```python
from build123d import *

# Parameters (mm, degrees)
BOSS_EXTRU_1_DEPTH      = 600
ESQUISSE2_R             = 15
ENL_V_MAT_EXTRU_1_DEPTH = 607.630035524


with BuildPart() as part:
    # Esquisse1 → Boss.-Extru.1 (new body)
    with BuildSketch(Plane.XY):
        with BuildLine():
            Line((2, -2), (78, -2))
            ThreePointArc((78, -2), (79.414213562, -1.414213562), (80, 0))
            Line((80, 0), (80, 36))
            ThreePointArc((80, 36), (79.414213562, 37.414213562), (78, 38))
            Line((78, 38), (2, 38))
            ThreePointArc((2, 38), (0.585786438, 37.414213562), (0, 36))
            Line((0, 36), (0, 0))
            ThreePointArc((0, 0), (0.585786438, -1.414213562), (2, -2))
        make_face()
        with BuildLine():
            Line((4, 4), (4, 32))
            ThreePointArc((4, 32), (4.585786438, 33.414213562), (6, 34))
            Line((6, 34), (74, 34))
            ThreePointArc((74, 34), (75.414213562, 33.414213562), (76, 32))
            Line((76, 32), (76, 4))
            ThreePointArc((76, 4), (75.414213562, 2.585786438), (74, 2))
            Line((74, 2), (6, 2))
            ThreePointArc((6, 2), (4.585786438, 2.585786438), (4, 4))
        make_face(mode=Mode.SUBTRACT)
    extrude(amount=BOSS_EXTRU_1_DEPTH)

    # Esquisse2 → Enlèv. mat.-Extru.1 (cut, through all)
    with BuildSketch(Plane(origin=(0, 38, 0), x_dir=(1, 0, 0), z_dir=(0, 1, 0))):
        with Locations(Location((40, -300, 0), (0, 0, 180))):
            Circle(ESQUISSE2_R)
    extrude(amount=-ENL_V_MAT_EXTRU_1_DEPTH, mode=Mode.SUBTRACT)


solid = part.part
```
Could you check a few things on this model? Use its own coordinates, in mm. A direction names the side the tool comes from. Round coordinates to 2 decimals unless told otherwise and drop trailing zeros. Write each loop counter-clockwise with the first axis right and the second up, starting at its lowest first coordinate (ties: lowest second). Pieces come first, ordered by that corner, then holes.
(1) Suppose I cut it at B-B on z = 300. Write out the boundary of the cut face in (x, y), and give its area (3 significant figures).
Findings below:
outline: (0, 0) arc R2 ccw to (2, -2) - (25, -2) - (25, 2) - (6, 2) arc R2 cw to (4, 4) - (4, 32) arc R2 cw to (6, 34) - (25, 34) - (25, 38) - (2, 38) arc R2 ccw to (0, 36) - close; (55, -2) - (78, -2) arc R2 ccw to (80, 0) - (80, 36) arc R2 ccw to (78, 38) - (55, 38) - (55, 34) - (74, 34) arc R2 cw to (76, 32) - (76, 4) arc R2 cw to (74, 2) - (55, 2) - close
area: 656 mm2
(2) Suppose I cut it at A-A on y = 25.5. Write out the boundary of the cut face in (x, z).
Findings below:
outline: (0, 0) - (4, 0) - (4, 600) - (0, 600) - close; (76, 0) - (80, 0) - (80, 600) - (76, 600) - close
(3) Thinking about a two-plate mould opening in Y: for faces 1 (the face through (23, -2, 296)), 2 (the face through (24, 38, 296)), 3 (the face through (41.953, 0.028, 314.872)), 4 (the face through (55, 34, 296)), which applies, +Y half, -Y half, draft (parallel to the pull), parting line (faces both ways), or undercut?
Findings below:
face 1: -Y half
face 2: +Y half
face 3: draft
face 4: undercut
(4) Suppose I cut it at D-D on z = 52.5. Write out the boundary of the cut face in (x, y), and give its area (3 significant figures).
Findings below:
outline: (0, 0) arc R2 ccw to (2, -2) - (78, -2) arc R2 ccw to (80, 0) - (80, 36) arc R2 ccw to (78, 38) - (2, 38) arc R2 ccw to (0, 36) - close; hole (4, 4) arc R2 ccw to (6, 2) - (74, 2) arc R2 ccw to (76, 4) - (76, 32) arc R2 ccw to (74, 34) - (6, 34) arc R2 ccw to (4, 32) - close
area: 896 mm2
(5) Which directions (+Z, -Z, +X, -X, +Y, -Y) give clear straight access to the entire face, cutting with the end or side of a thin tool? Please do faces 5 (the face through (36.9, 1.8, 0)), 6 (the face through (4, 18, 296)).
Findings below:
face 5: -Z, +X, -X, +Y, -Y
face 6: +Z, -Z
(6) If I drill on probe 1 along Y at (x, z) = (25.5, 236.5); probe 2 along X at (y, z) = (18.5, 475); probe 3 along Z at (x, y) = (40, 0), over which ranges is the centre line in solid material (lowest first)?
Findings below:
probe 1: y = -2 to 2, 34 to 38
probe 2: x = 0 to 4, 76 to 80
probe 3: z = 0 to 285, 315 to 600
(7) Suppose I cut it at C-C on x = 17. Write out the boundary of the cut face in (y, z), and give its area (3 significant figures).
Findings below:
outline: (-2, 0) - (2, 0) - (2, 600) - (-2, 600) - close; (34, 0) - (38, 0) - (38, 600) - (34, 600) - close
area: 4,800 mm2
